from build123d import *

# Parameters (mm, degrees)
SKETCH1_R           = 25
BOSS_EXTRUDE1_DEPTH = 50
SKETCH4_W           = 5
SKETCH4_H           = 13
SKETCH2_R           = 22
CUT_EXTRUDE1_DEPTH  = 74.402997214
CUT_EXTRUDE1_DRAFT  = -5
SKETCH3_R           = 22
CUT_EXTRUDE2_DEPTH  = 30


with BuildPart() as part:
    # Sketch1 → Boss-Extrude1 (new body)
    with BuildSketch(Plane.XY):
        Circle(SKETCH1_R)
    extrude(amount=BOSS_EXTRUDE1_DEPTH)

    # Sketch4 → Revolve1 (revolve)
    with BuildSketch(Plane(origin=(0, 0, 0), x_dir=(0, 0, -1), z_dir=(1, 0, 0)), mode=Mode.PRIVATE) as revolve1_sk:
        with Locations((-2.5, 31.5)):
            Rectangle(SKETCH4_W, SKETCH4_H)
    revolve(revolve1_sk.sketch.rotate(Axis((0, 0, -2.5), (0, 0, 1)), 90), axis=Axis((0, 0, -2.5), (0, 0, 1)))


with BuildPart() as cut_extrude1_tool:
    # Sketch2 → Cut-Extrude1 (with draft: the straight prism first)
    with BuildSketch(Plane(origin=(0, 0, 0), x_dir=(-1, 0, 0), z_dir=(0, 0, -1))):
        Circle(SKETCH2_R)
    extrude(amount=-CUT_EXTRUDE1_DEPTH)
    # Cut-Extrude1: the draft: its side faces are tilted about the plane it starts from
    cut_extrude1_sides = [cut_extrude1_tool.faces().sort_by_distance(p)[0] for p in [
        (22, 0, 37.201498607),
    ]]
    draft(cut_extrude1_sides, Plane(origin=(0, 0, 0), x_dir=(-1, 0, 0), z_dir=(0, 0, -1)), CUT_EXTRUDE1_DRAFT)


with BuildPart() as part_1:
    add(part.part)

    # Cut-Extrude1: cut by cut_extrude1_tool
    add(cut_extrude1_tool.part, mode=Mode.SUBTRACT)

    # Sketch3 → Cut-Extrude2 (cut)
    with BuildSketch(Plane.XY.offset(50)):
        Circle(SKETCH3_R)
    extrude(amount=-CUT_EXTRUDE2_DEPTH, mode=Mode.SUBTRACT)


solid = part_1.part
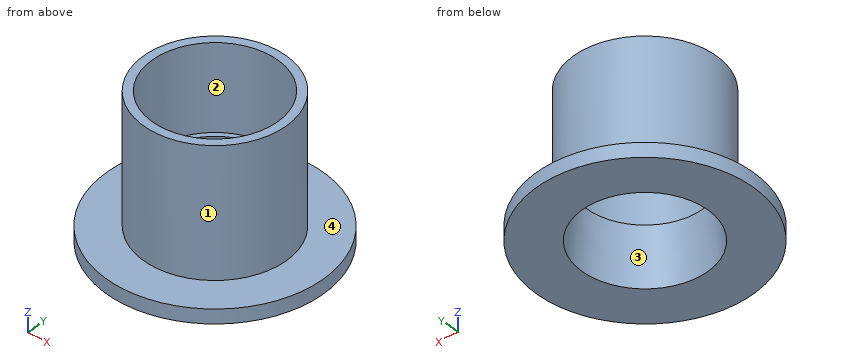
For this review, take the finished solid that the model builds, in its own axes (mm). Face numbers are marked on the shaded views. Coordinates: 2 decimals unless noted, no trailing zeros. Order: outer loops, then holes, each group sorted by start corner. A loop starts at its lowest first (then second) coordinate and runs counter-clockwise, first axis right, second up. Notation, with made-up numbers: (-7, -1) - (48, -1) arc R23 ccw to (48, 22) - close; hole circle Ø4 at (-26.75, 76). An arc over 180 degrees is marked (long way). Answer as CSV lines item,"result". Start each with the question number.
1) Draft analysis for pull direction Y (two halves, no side actions). For the marked faces 1, 2, 3 and 4, state which applies: +Y half, -Y half, draft (parallel to the pull), parting line (faces both ways), or undercut.
2) To check wall thickness, follow line 1 along Y through (x, z) = (-1, 37.5); line 2 along Z through (x, y) = (11, -23); line 3 along Y through (x, z) = (7.5, 30). State the ranges of each line that lie inside material, in increasing order. Write a range as [from, to].
3) Add section D-D (y = -31). State the section outline as (x, z) points.
4) Insertion check: P1, Ø8, axis at y = -1.5, z = 35, coming from the +X side; P2, Ø8, axis at x = 25, z = 33.5, coming from the -Y side; P3, Ø12, axis at x = 15.5, y = -7, coming from the +Z side; P4, Ø5, axis at y = -22, z = 38.5, coming from the +X side. Each pin has a flat end and moves straight along its axis. Give the tip position at first contact, or say it passes through.
5) Add section A-A (y = 0). State the section outline as (x, z) points, then the cut area to 3 significant figures.
6) Add section C-C (z = 35). State the section outline as (x, y) points, then the cut area to 3 significant figures.
Result:
1,face 1,"parting line"
1,face 2,"undercut"
1,face 3,"undercut"
1,face 4,"draft"
2,line 1,"[-24.98, -21.98], [21.98, 24.98]"
2,line 2,"[0, 5]"
2,line 3,"[-23.85, -20.68], [20.68, 23.85]"
3,outline,"(-21.98, 0) - (21.98, 0) - (21.98, 5) - (-21.98, 5) - close"
4,P1,"x = 25"
4,P2,"y = -13.56"
4,P3,"z = 50"
4,P4,"x = 15.64"
5,outline,"(-38, 0) - (-22, 0) - (-20.25, 20) - (-22, 20) - (-22, 50) - (-25, 50) - (-25, 5) - (-38, 5) - close; (20.25, 20) - (22, 0) - (38, 0) - (38, 5) - (25, 5) - (25, 50) - (22, 50) - (22, 20) - close"
5,area,"465 mm^2"
6,outline,"circle Ø50 at (0, 0); hole circle Ø44 at (0, 0)"
6,area,"443 mm^2"
